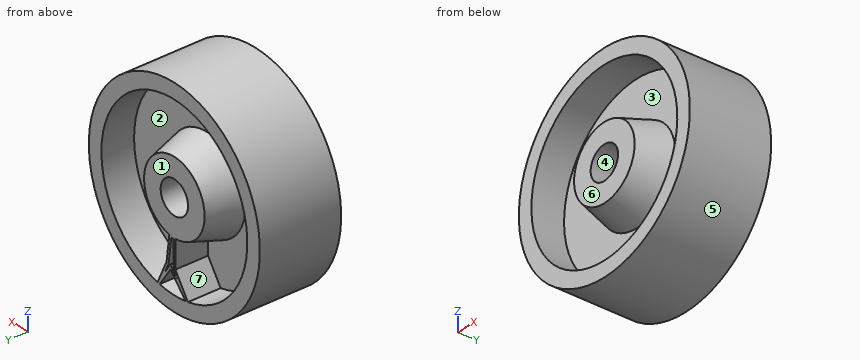
```python
from build123d import *

# Parameters (mm, degrees)
RIB3_REACH = 849.461


with BuildPart() as part:
    # Sketch2 → Revolve2 (revolve)
    with BuildSketch(Plane.XY, mode=Mode.PRIVATE) as revolve2_sk:
        Polygon((-83.825932003, -205.951906896), (-83.825932003, 205.951906896), (-185.425932003, 205.951906896), (-234.75772391, 40.338034064), (-446.766972465, 40.338034064), (-446.766972465, 205.951906896), (-523.701076512, 205.951906896), (-523.701076512, -205.951906896), (-446.766972465, -205.951906896), (-446.766972465, -40.338034064), (-234.75772391, -40.338034064), (-185.425932003, -205.951906896), align=None)
    revolve(revolve2_sk.sketch.rotate(Axis((0, 0, 0), (0, 1, 0)), 270), axis=Axis((0, 0, 0), (0, 1, 0)))

    # Sketch15 walls → Rib3 (add, up to next)
    with BuildSketch(Plane(origin=(0, 205.951906896, 0), x_dir=(1, 0, 0), z_dir=(0, 1, 0)), mode=Mode.PRIVATE) as rib3_sk1:
        Polygon((-6.35, 179.47656005), (-6.35, 326.47470397), (-135.682333379, 515.555894782), (23.333889095, 338.748721611), (135.129805155, 505.477172887), (47.662469422, 314.977908793), (29.606309095, 177.131658856), align=None)
        Polygon((6.35, 191.375303956), (6.35, 330.402645947), (-17.181459102, 364.805151432), (24.798310455, 318.128628306), (57.585986403, 367.02700156), (35.319488971, 318.531739424), (18.559266197, 190.579073097), align=None, mode=Mode.SUBTRACT)
    rib3_tool1 = extrude(rib3_sk1.sketch, amount=-RIB3_REACH, mode=Mode.PRIVATE) - part.part
    add(rib3_tool1.solids().sort_by_distance((60.211997777, 205.951906896, -382.345381091))[0])


solid = part.part
```
The listing builds one solid part. Answer for the finished solid, in the listing's coordinates (mm). Face numbers are marked on the shaded views. A direction names the side the tool comes from. Round coordinates to 2 decimals unless told otherwise and drop trailing zeros. Loops run counter-clockwise (first coordinate to the right, second up) from the corner with the lowest first, then second, coordinate; pieces in that order, holes last.
Q1. Section A-A, the plane z = 0 is taken. Determine the outline of the cut face in (x, y).
Q2. Section D-D, the plane y = 159 is taken. Determine the outline of the cut face in (x, z).
Q3. Given pin 1 Ø6 at (x, y) = (274.5, -120) entering from -Z; pin 2 Ø6 at (x, z) = (389.5, 358.5) entering from +Y; pin 3 Ø10 at (x, y) = (55, 153.5) entering from +Z; pin 4 Ø2 at (x, y) = (-141.5, 86.5) entering from +Z, each flat-ended and moving along its own axis, determine where each tip first touches the part or whether it passes through.
Q4. For a pull along Z with two mould halves and no side action, classify the marked faces 4, 5, 6 and 7 as released by +Z, released by -Z, zero draft, split by the parting line, or undercut.
Q5. Which of the six approach directions +Z, -Z, +X, -X, +Y, -Y give full straight-line access (tool end or side, diameter ignored) to the marked faces 1, 2 and 3?
Q6. Section B-B, the plane y = -142 is taken. Determine the outline of the cut face in (x, z).
Q7. Find the intervals of material crossed by line 1 (X direction, y = 73, z = 0); line 2 (X direction, y = 89, z = 0); line 3 (Z direction, x = 29, y = -186), in increasing order.
Q8. Section C-C, the plane x = 274 is taken. Determine the outline of the cut face in (y, z).
Completed:
1. outline: (-523.7, -205.95) - (-446.77, -205.95) - (-446.77, -40.34) - (-234.76, -40.34) - (-185.43, -205.95) - (-83.83, -205.95) - (-83.83, 205.95) - (-185.43, 205.95) - (-234.76, 40.34) - (-446.77, 40.34) - (-446.77, 205.95) - (-523.7, 205.95) - close; (83.83, -205.95) - (185.43, -205.95) - (234.76, -40.34) - (446.77, -40.34) - (446.77, -205.95) - (523.7, -205.95) - (523.7, 205.95) - (446.77, 205.95) - (446.77, 40.34) - (234.76, 40.34) - (185.43, 205.95) - (83.83, 205.95) - close
2. outline: circle Ø1047.4 at (0, 0); hole circle Ø167.65 at (0, 0); hole (-83.27, -438.94) - (-6.35, -326.47) - (-6.35, -199.31) arc R199.41 cw (long way) to (32.18, -196.8) - (47.66, -314.98) - (102.68, -434.81) arc R446.77 ccw (long way) to start; hole (-68.99, -441.41) arc R446.77 ccw to (89.67, -437.68) - (23.33, -338.75) - close; hole (-17.18, -364.81) - (24.8, -318.13) - (57.59, -367.03) - (35.32, -318.53) - (19.59, -198.45) arc R199.41 cw to (6.35, -199.31) - (6.35, -330.4) - close
3. pin 1: stops at z = -447.83
3. pin 2: passes through
3. pin 3: stops at z = 521.31
3. pin 4: stops at z = 504.5
4. face 4: undercut
4. face 5: split by the parting line
4. face 6: zero draft
4. face 7: undercut
5. face 1: +Z, -Z, +X, -X, +Y
5. face 2: +Y
5. face 3: -Y
6. outline: circle Ø1047.4 at (0, 0); circle Ø408.95 at (0, 0); hole circle Ø893.53 at (0, 0); hole circle Ø167.65 at (0, 0)
7. line 1: x = -523.7 to -446.77, -225.03 to -83.83, 83.83 to 225.03, 446.77 to 523.7
7. line 2: x = -523.7 to -446.77, -220.26 to -83.83, 83.83 to 220.26, 446.77 to 523.7
7. line 3: z = -522.9 to -445.82, -189.16 to -78.65, 78.65 to 189.16, 445.82 to 522.9
8. outline: (-205.95, -446.3) - (205.95, -446.3) - (205.95, -352.88) - (40.34, -352.88) - (40.34, 352.88) - (205.95, 352.88) - (205.95, 446.3) - (-205.95, 446.3) - (-205.95, 352.88) - (-40.34, 352.88) - (-40.34, -352.88) - (-205.95, -352.88) - close
